```python
from build123d import *

# Parameters (mm, degrees)
SKETCH1_W                = 70
SKETCH1_H                = 50
BOSS_EXTRUDE1_DEPTH      = 30
SKETCH2_W                = 61.1
SKETCH2_H                = 43.3
CUT_EXTRUDE1_DEPTH       = 28
CUT_EXTRUDE1_DRAFT       = -2
SKETCH3_W                = 7
SKETCH3_H                = 13.35
HANG_TABS_DEPTH          = 30
BOSS_EXTRUDE3_DEPTH      = 12
BOSS_EXTRUDE3_DEPTH_BACK = 15
SKETCH5_R                = 1.5
CUT_EXTRUDE2_DEPTH       = 15
SKETCH6_R                = 5
CUT_EXTRUDE3_DEPTH       = 58.879184514
CUT_EXTRUDE4_DEPTH       = 58.879184514
CUT_EXTRUDE5_START       = -28
SKETCH8_R                = 2.5
CUT_EXTRUDE5_DEPTH       = 30.879184514
CUT_EXTRUDE6_START       = 28
SKETCH8_2_R              = 2.5
CUT_EXTRUDE6_DEPTH       = 30.879184514
FILLET2_R                = 5
FILLET3_R                = 5
CHAMFER1_SIZE            = 5
FILLET4_R                = 5
BOSS_EXTRUDE4_START      = -17.5
SKETCH9_W                = 15
SKETCH9_H                = 5
BOSS_EXTRUDE4_DEPTH      = 10.5
FILLET5_R                = 5
FILLET6_R                = 1


with BuildPart() as part:
    # Sketch1 → Boss-Extrude1 (new body)
    with BuildSketch(Plane(origin=(0, 0, 0), x_dir=(0, 0, -1), z_dir=(1, 0, 0))):
        Rectangle(SKETCH1_W, SKETCH1_H)
    extrude(amount=BOSS_EXTRUDE1_DEPTH)


with BuildPart() as cut_extrude1_tool:
    # Sketch2 → Cut-Extrude1 (with draft: the straight prism first)
    with BuildSketch(Plane.ZY):
        Rectangle(SKETCH2_W, SKETCH2_H)
    extrude(amount=-CUT_EXTRUDE1_DEPTH)
    # Cut-Extrude1: the draft: its side faces are tilted about the plane it starts from
    cut_extrude1_sides = [cut_extrude1_tool.faces().sort_by_distance(p)[0] for p in [
        (14, -21.65, 0),
        (14, 0, 30.55),
        (14, 21.65, 0),
        (14, 0, -30.55),
    ]]
    draft(cut_extrude1_sides, Plane.ZY, CUT_EXTRUDE1_DRAFT)


with BuildPart() as part_1:
    add(part.part)

    # Cut-Extrude1: cut by cut_extrude1_tool
    add(cut_extrude1_tool.part, mode=Mode.SUBTRACT)

    # Sketch3 → Hang tabs (add)
    with BuildSketch(Plane(origin=(0, 0, 0), x_dir=(0, 0, -1), z_dir=(1, 0, 0))):
        with Locations((-31.5, 28.325)):
            Rectangle(SKETCH3_W, SKETCH3_H)
        with Locations((31.5, 28.325)):
            Rectangle(SKETCH3_W, SKETCH3_H)
    extrude(amount=HANG_TABS_DEPTH)

    # Sketch4 → Boss-Extrude3 (add, two sides: drawn at the far end of the back side and taken through both)
    with BuildSketch(Plane.ZY.offset(-BOSS_EXTRUDE3_DEPTH_BACK)):
        with BuildLine():
            Line((-6, 25), (-6, 21.65))
            Line((-6, 21.65), (6, 21.65))
            Line((6, 21.65), (6, 25))
            ThreePointArc((6, 25), (0, 31), (-6, 25))
        make_face()
        with BuildLine():
            Line((-6, -21.65), (6, -21.65))
            Line((6, -21.65), (6, -25))
            ThreePointArc((6, -25), (0, -31), (-6, -25))
            Line((-6, -25), (-6, -21.65))
        make_face()
    extrude(amount=BOSS_EXTRUDE3_DEPTH + BOSS_EXTRUDE3_DEPTH_BACK)

    # Sketch5 → Cut-Extrude2 (cut)
    with BuildSketch(Plane.ZY.offset(12)):
        with Locations((0, 25)):
            Circle(SKETCH5_R)
        with Locations((0, -25)):
            Circle(SKETCH5_R)
    extrude(amount=-CUT_EXTRUDE2_DEPTH, mode=Mode.SUBTRACT)

    # Sketch6 → Cut-Extrude3 (cut, through all)
    with BuildSketch(Plane(origin=(0, 0, 0), x_dir=(1, 0, 0), z_dir=(0, 1, 0))):
        with Locations((0, 17.55)):
            Circle(SKETCH6_R)
    extrude(amount=CUT_EXTRUDE3_DEPTH, mode=Mode.SUBTRACT)

    # Sketch7 → Cut-Extrude4 (cut, through all)
    with BuildSketch(Plane(origin=(0, 0, 0), x_dir=(1, 0, 0), z_dir=(0, 1, 0))):
        with BuildLine():
            Line((6, -19), (6, -23))
            ThreePointArc((6, -23), (4, -25), (2, -23))
            Line((2, -23), (2, -19))
            ThreePointArc((2, -19), (4, -17), (6, -19))
        make_face()
    extrude(amount=CUT_EXTRUDE4_DEPTH, mode=Mode.SUBTRACT)

    # Sketch8 → Cut-Extrude5 (cut, through all)
    with BuildSketch(Plane.XY.offset(CUT_EXTRUDE5_START)):
        with Locations((15, 30)):
            Circle(SKETCH8_R)
        with Locations((22.5, 30)):
            Circle(SKETCH8_R)
        with Locations((7.5, 30)):
            Circle(SKETCH8_R)
    extrude(amount=-CUT_EXTRUDE5_DEPTH, mode=Mode.SUBTRACT)

    # Sketch8<2> → Cut-Extrude6 (cut, through all)
    with BuildSketch(Plane.XY.offset(CUT_EXTRUDE6_START)):
        with Locations((15, 30)):
            Circle(SKETCH8_2_R)
        with Locations((22.5, 30)):
            Circle(SKETCH8_2_R)
        with Locations((7.5, 30)):
            Circle(SKETCH8_2_R)
    extrude(amount=CUT_EXTRUDE6_DEPTH, mode=Mode.SUBTRACT)

    # Fillet2
    fillet2_edges = [part_1.edges().sort_by_distance(p)[0] for p in [
        (30, 35, 31.5),
        (0, 35, 31.5),
        (30, 35, -31.5),
        (0, 35, -31.5),
    ]]
    fillet(fillet2_edges, radius=FILLET2_R)

    # Fillet3
    fillet3_edges = [part_1.edges().sort_by_distance(p)[0] for p in [
        (15, 31, 0),
        (15, -31, 0),
    ]]
    fillet(fillet3_edges, radius=FILLET3_R)

    # Chamfer1
    # the kernel refuses this chamfer: 5 mm, written as the material it takes off along each edge
    with BuildSketch(Plane(origin=(0, 25, -17.55), x_dir=(-0.9999950652018581, 0, -0.003141587485879425), z_dir=(-0.003141587485879425, 0, 0.9999950652018581))) as chamfer1_piece_1:
        Polygon((5 + CHAMFER1_SIZE, 0), (5, CHAMFER1_SIZE), (5, 0), align=None)
    revolve(axis=Axis((0, 25, -17.55), (0, -1, 0)), revolution_arc=359.64, mode=Mode.SUBTRACT)

    # Fillet4
    fillet4_edges = [part_1.edges().sort_by_distance(p)[0] for p in [
        (15, -25, -35),
        (15, -25, 35),
    ]]
    fillet(fillet4_edges, radius=FILLET4_R)

    # Sketch9 → Boss-Extrude4 (add)
    with BuildSketch(Plane.ZY.offset(BOSS_EXTRUDE4_START)):
        with Locations((0, 19.15)):
            Rectangle(SKETCH9_W, SKETCH9_H)
        with Locations((0, -19.15)):
            Rectangle(SKETCH9_W, SKETCH9_H)
    extrude(amount=-BOSS_EXTRUDE4_DEPTH)

    # Fillet5
    fillet5_edges = [part_1.edges().sort_by_distance(p)[0] for p in [
        (0, 23.325, 6),
        (0, -23.325, 6),
        (0, -23.325, -6),
    ]]
    fillet(fillet5_edges, radius=FILLET5_R)

    # Fillet6
    fillet6_edges = [part_1.edges().sort_by_distance(p)[0] for p in [
        (14, 21.161109227, 30.061109227),
        (14, -21.161109227, 30.061109227),
        (14, -21.161109227, -30.061109227),
        (14, 21.161109227, -30.061109227),
        (28, 0, 29.572218454),
        (28, -20.672218454, 18.536109227),
        (28, 0, -29.572218454),
        (28, 20.672218454, -18.536109227),
        (28, 20.672218454, 18.536109227),
        (28, -20.672218454, -18.536109227),
    ]]
    fillet(fillet6_edges, radius=FILLET6_R)


solid = part_1.part
```
Can you work these out from the model? Positions are in its coordinate system, mm. A direction names the side the tool comes from. Coordinates: 2 decimals unless noted, no trailing zeros. Write each loop counter-clockwise with the first axis right and the second up, starting at its lowest first coordinate (ties: lowest second). Pieces come first, ordered by that corner, then holes. Notation, with made-up numbers: (61.25, 57.25) - (120.25, 57.25) arc R16 ccw to (120.25, 83.25) - close; hole circle Ø5 at (-25, 47). An arc over 180 degrees is marked (long way). Return JSON: item names as keys, results as strings.
Q1. I'm going to push flat-ended pins straight in: pin 1 Ø0.5 at (y, z) = (-25.5, 0.5) entering from +X; pin 2 Ø8 at (y, z) = (-9, 5.5) entering from -X; pin 3 Ø4 at (y, z) = (22.5, 20.5) entering from -X. Where does each tip first touch, or does it pass through?
Computed values:
{"pin 1": "stops at x = 15", "pin 2": "stops at x = 28", "pin 3": "stops at x = 0"}
Q2. If we section it at D-D (x = 22.5): Count the separate pieces of the cut face and the enclosed holes in it, then the cut area to 3 significant figures.
Computed values:
{"separate pieces": "3", "enclosed holes": "1", "area": "1,200 mm2"}
Q3. Please list where these lines run through material, in increasing order: L1, parallel to Y at x = -4, z = 0; L2, parallel to X at y = 30, z = 31; L3, parallel to Y at x = 18, z = 16.5. Write a range as from..to.
Computed values:
{"L1": "y = -31..-26.5, -23.5..-21.65, 21.65..23.5, 26.5..31", "L2": "x = 0..5, 10..12.5, 17.5..20, 25..30", "L3": "y = -25..-21.02, 21.02..25"}
Q4. On a 3-axis mill with a long thin cutter (end or side, diameter ignored), from which of +Z, -Z, +X, -X, +Y, -Y can I reach the whole of each face in a straight line? I mean faces 1 (the flat face through (23, -19, -7.5)), 2 (the flat face through (15, 27, -28)), 3 (the cylindrical face through (9, 32, -31)), 4 (the cylindrical face through (9, 32, 31)). Say none if no direction works.
Computed values:
{"face 1": "-X", "face 2": "+X, -X, +Y", "face 3": "-Z", "face 4": "+Z"}
Q5. If we section it at C-C (z = 10): Please give me the cut outline in (x, y), then the cut area to 3 significant figures.
Computed values:
{"outline": "(-0.1, -25) - (30, -25) - (30, 25) - (-0.1, 25) - (-0.1, 21.65) - (0, 21.65) - (27.03, 20.71) arc R1 cw to (28, 19.71) - (28, -19.71) arc R1 cw to (27.03, -20.71) - (0, -21.65) - (-0.1, -21.65) - close", "area": "316 mm2"}
Q6. If we section it at A-A (x = -8): Please give me the cut outline in (y, z).
Computed values:
{"outline": "(-25, -6) - (-21.65, -6) - (-21.65, 6) - (-25, 6) arc R6 ccw to start; (21.65, -6) - (25, -6) arc R6 ccw to (25, 6) - (21.65, 6) - close; hole circle Ø3 at (-25, 0); hole circle Ø3 at (25, 0)"}
Q7. If we section it at B-B (y = -6): Please give me the cut outline in (x, z), then the cut area to 3 significant figures.
Computed values:
{"outline": "(0, -35) - (30, -35) - (30, 35) - (0, 35) - (0, 30.55) - (27.03, 29.61) arc R1 cw to (28, 28.61) - (28, -28.61) arc R1 cw to (27.03, -29.61) - (0, -30.55) - close", "area": "417 mm2"}
Q8. Thinking about a two-plate mould opening in Y: for faces 5 (the conical face through (6.6, 21.6, -17.7)), 6 (the cylindrical face through (13.711, -20.886, -29.771)), 7 (the cylindrical face through (-1, 23, 8)), which applies, +Y half, -Y half, draft (parallel to the pull), parting line (faces both ways), or undercut?
Computed values:
{"face 5": "+Y half", "face 6": "undercut", "face 7": "draft"}
